from build123d import *

# Parameters (mm, degrees)
RESSALTO_EXTRUS_O1_DEPTH = 20
ESBO_O2_W                = 2
ESBO_O2_H                = 30
RESSALTO_EXTRUS_O2_DEPTH = 60
RESSALTO_EXTRUS_O3_DEPTH = 8
FILETE1_R                = 1
ESBO_O4_R                = 1.5
CORTE_EXTRUS_O1_DEPTH    = 8
CHANFRO1_SIZE            = 19
FILETE2_R                = 3
FILETE3_R                = 1


with BuildPart() as part:
    # Esboço1 → Ressalto-extrusão1 (new body)
    with BuildSketch(Plane.XY):
        Polygon((-4.205798406, -35.280489631), (-4.205798406, 34.719510369), (8.794201594, 34.719510369), (8.794201594, 31.719510369), (11.794201594, 31.719510369), (11.794201594, 36.719510369), (-6.205798406, 36.719510369), (-6.205798406, -37.280489631), (11.794201594, -37.280489631), (11.794201594, -32.280489631), (8.794201594, -32.280489631), (8.794201594, -35.280489631), align=None)
    extrude(amount=RESSALTO_EXTRUS_O1_DEPTH)

    # Esboço2 → Ressalto-extrusão2 (add)
    with BuildSketch(Plane(origin=(0, 0, 0), x_dir=(-1, 0, 0), z_dir=(0, 0, -1))):
        with Locations((5.205798406, 0)):
            Rectangle(ESBO_O2_W, ESBO_O2_H)
    extrude(amount=RESSALTO_EXTRUS_O2_DEPTH)

    # Esboço3 → Ressalto-extrusão3 (add)
    with BuildSketch(Plane(origin=(0, 15, 0), x_dir=(1, 0, 0), z_dir=(0, 1, 0))):
        Polygon((-6.205798406, 60), (-6.205798406, 63), (11.794201594, 63), (11.794201594, 57), (8.794201594, 57), (8.794201594, 60), align=None)
    ressalto_extrus_o3 = extrude(amount=-RESSALTO_EXTRUS_O3_DEPTH)

    # Espelhar1: Ressalto-extrusão3 across plane
    add(ressalto_extrus_o3.mirror(Plane.ZX))

    # Filete1
    filete1_edges = [part.edges().sort_by_distance(p)[0] for p in [
        (-4.205798406, 34.719510369, 10),
        (-4.205798406, -35.280489631, 10),
        (11.794201594, -37.280489631, 10),
        (11.794201594, 36.719510369, 10),
        (-4.205798406, 11, -60),
        (11.794201594, 11, -63),
        (11.794201594, 11, -57),
        (-4.205798406, -11, -60),
        (11.794201594, -11, -57),
        (11.794201594, -11, -63),
    ]]
    fillet(filete1_edges, radius=FILETE1_R)

    # Esboço4 → Corte-extrusão1 (cut)
    with BuildSketch(Plane(origin=(-4.205798406, 0, 0), x_dir=(0, 0, -1), z_dir=(1, 0, 0))):
        with Locations(Location((-10, -0.140244815, 0), (0, 0, 90))):
            Circle(ESBO_O4_R)
    extrude(amount=-CORTE_EXTRUS_O1_DEPTH, mode=Mode.SUBTRACT)

    # Chanfro1
    chanfro1_edges = [part.edges().sort_by_distance(p)[0] for p in [
        (-5.205798406, -15, 0),
        (-5.205798406, 15, 0),
    ]]
    chamfer(chanfro1_edges, length=CHANFRO1_SIZE)

    # Filete2
    filete2_edges = [part.edges().sort_by_distance(p)[0] for p in [
        (-5.205798406, -15, -19),
        (-5.205798406, 15, -19),
    ]]
    fillet(filete2_edges, radius=FILETE2_R)

    # Filete3
    filete3_edges = [part.edges().sort_by_distance(p)[0] for p in [
        (-5.205798406, -34, 0),
        (-5.185726934, 34, 0),
    ]]
    fillet(filete3_edges, radius=FILETE3_R)


solid = part.part
Check sheet for the modelled part. Datum: model origin and axes. Units: mm. A direction names the side the tool comes from. Round coordinates to 2 decimals unless told otherwise and drop trailing zeros. Order: outer loops, then holes, each group sorted by start corner. A loop starts at its lowest first (then second) coordinate and runs counter-clockwise, first axis right, second up.
(1) Access from +Z, -Z, +X, -X, +Y, -Y to the whole of each face (thin tool, end or side, straight path). Record for faces 1 (the flat face through (10, -11, -57)), 2 (the flat face through (3, 11, -60)), 3 (the flat face through (10, -32.28, 10)), 4 (the cylindrical face through (-5.22, 15.22, -19.11)), 5 (the flat face through (-5, -25, -9)).
(2) Scan lines: probe 1 along Y at (x, z) = (8.25, 17); probe 2 along Y at (x, z) = (10.25, 9); probe 3 along Z at (x, y) = (1.75, -10). Record each from-to range of solid material in increasing order.
(3) Draft check along X on faces 6 (the flat face through (8.794, 33, 10)), 7 (the flat face through (-6.206, -1, -12)), 8 (the flat face through (8.794, -11, -58)), 9 (the cylindrical face through (-5.192, -0.465, 8.536)). Enter one of: pulls with the +X half, pulls with the -X half, needs draft (parallel to the pull), parting line crosses it, or undercut.
(4) Cross-section at B-B, the plane z = 10. Enter the section's corners in (x, y), and give its area (3 significant figures).
(5) Cross-section at A-A, the plane x = 0.5. Enter the section's corners in (y, z), and give its area (3 significant figures).
(6) Cross-section at D-D, the plane z = -8. Enter the section's corners in (x, y).
(7) Go/stop test with flat-tipped pins: P1, Ø1, axis at x = 9.5, y = 11.5, coming from the +Z side; P2, Ø1.6, axis at x = -5, y = 0.5, coming from the -Z side; P3, Ø6, axis at y = 7, z = 6, coming from the +X side; P4, Ø1.8, axis at y = -0.14, z = 10, coming from the -X side. Record where each tip stops, or that it passes through.
(8) Cross-section at C-C, the plane y = 8. Enter the section's corners in (x, z), and give its area (3 significant figures).
Check sheet entries:
1. face 1: +Z, +X, +Y, -Y
1. face 2: +Z, +Y, -Y
1. face 3: +Z, -Z, +X
1. face 4: -Z, +X, -X, +Y
1. face 5: -Z, +X, -X, -Y
2. probe 1: y = -37.28 to -35.28, 34.72 to 36.72
2. probe 2: y = -37.28 to -32.28, 31.72 to 36.72
2. probe 3: z = -63 to -60
3. face 6: undercut
3. face 7: pulls with the -X half
3. face 8: undercut
3. face 9: needs draft
4. outline: (-6.21, -37.28) - (10.79, -37.28) arc R1 ccw to (11.79, -36.28) - (11.79, -32.28) - (8.79, -32.28) - (8.79, -35.28) - (-3.21, -35.28) arc R1 cw to (-4.21, -34.28) - (-4.21, -1.64) - (-6.21, -1.64) - close; (-6.21, 1.36) - (-4.21, 1.36) - (-4.21, 33.72) arc R1 cw to (-3.21, 34.72) - (8.79, 34.72) - (8.79, 31.72) - (11.79, 31.72) - (11.79, 35.72) arc R1 ccw to (10.79, 36.72) - (-6.21, 36.72) - close
4. area: 224 mm2
5. outline: (-37.28, 0) - (-35.28, 0) - (-35.28, 20) - (-37.28, 20) - close; (-15, -63) - (-7, -63) - (-7, -60) - (-15, -60) - close; (7, -63) - (15, -63) - (15, -60) - (7, -60) - close; (34.72, 0) - (36.72, 0) - (36.72, 20) - (34.72, 20) - close
5. area: 128 mm2
6. outline: (-6.21, -26) - (-4.21, -26) - (-4.21, 26) - (-6.21, 26) - close
7. P1: stops at z = -57
7. P2: stops at z = -60
7. P3: stops at x = -4.21
7. P4: passes through
8. outline: (-6.21, -63) - (10.79, -63) arc R1 ccw to (11.79, -62) - (11.79, -58) arc R1 ccw to (10.79, -57) - (8.79, -57) - (8.79, -60) - (-3.21, -60) arc R1 cw to (-4.21, -59) - (-4.21, 20) - (-6.21, 20) - close
8. area: 223 mm2
